Check sheet for the modelled part. Datum: model origin and axes. Units: mm. A direction names the side the tool comes from. Give positions to 0.01 mm unless a question says otherwise; leave off trailing zeros. Write each loop counter-clockwise with the first axis right and the second up, starting at its lowest first coordinate (ties: lowest second). Pieces come first, ordered by that corner, then holes. Notation, with made-up numbers: M 4.5,-32.75 L 63.5,-32.75 A13 cw 63.5,-24.75 Z; hole C 37.5,-9.75 d5. An arc over 180 degrees is marked long. One line per item, written item: value. Start each with the question number.
from build123d import *

# Parameters (mm, degrees)
F1_DEPTH = 15
F2_W     = 50
F2_H     = 32
F3_DEPTH = 150
F4_T     = -2.5


with BuildPart() as f1:
    # F0 (on Top) → F1 (new body)
    with BuildSketch(Plane.XY):
        with BuildLine():
            Line((100, 50), (-100, 50))
            Line((-100, 50), (-100, -50))
            add(Edge.make_bspline(
                [(-100, -50), (-66.6666666667, -68.9898259938), (0, -106.9694779813), (66.6666666667, -68.9898259938), (100, -50)],
                knots=[0, 0, 0, 0, 0.5, 1, 1, 1, 1], degree=3))
            Line((100, -50), (100, 50))
        make_face()
    extrude(amount=F1_DEPTH)

    # F2 (on face) → F3 (join)
    with BuildSketch(Plane.XY.offset(15)):
        with Locations((0, 25.8605617276)):
            Rectangle(F2_W, F2_H)
    extrude(amount=F3_DEPTH)

    # F4
    f4_openings = [f1.faces().sort_by_distance(p)[0] for p in [
        (0, 25.860562, 165),
    ]]
    offset(amount=F4_T, openings=f4_openings, kind=Kind.INTERSECTION)


solid = f1.part
1) Tool access check on faces 1 (the flat face through (0, 39.361, 88)), 2 (the flat face through (-1, -18, 2.5)), 3 (the flat face through (-25, 26, 89)). Record the directions out of +Z, -Z, +X, -X, +Y, -Y that give a thin tool (end or side, any length) a straight path to the whole face; none if there is none.
2) Gauge pin test, flat ends, axial feed: pin 1 (22.5 mm diameter, centred on x = -6.5, z = 73, fed in from +Y); pin 2 (22.5 mm diameter, centred on x = -11, z = 123, fed in from -Y); pin 3 (5 mm diameter, centred on x = -65, y = -68.5, fed in from +Z). Record the tip position at first contact, or that the pin passes through.
3) Cross-section at A-A (z = 95). Record the boundary of the cut face in (x, y), plus the area to 3 significant figures.
4) Material ranges on L1, parallel to Z at x = -58.5, y = -18; L2, parallel to X at y = 36.5, z = 98.5; L3, parallel to X at y = 21.5, z = 11, recorded low to high. Write a range as from..to.
5) Draft check along Y on faces 4 (the flat face through (1, 50, 7)), 5 (the flat face through (25, 26, 89)), 6 (the flat face through (-22.5, 26, 88)), 7 (the flat face through (0, 9.861, 89)). Enter one of: released by +Y, released by -Y, zero draft, split by the parting line, or undercut.
6) Cross-section at B-B (y = 6.5). Record the boundary of the cut face in (x, z).
Data:
1. face 1: +Z
1. face 2: none
1. face 3: +Z, -X, +Y, -Y
2. pin 1: stops at y = 41.86
2. pin 2: stops at y = 9.86
2. pin 3: stops at z = 15
3. outline: M -25,9.86 L 25,9.86 L 25,41.86 L -25,41.86 Z; hole M -22.5,12.36 L 22.5,12.36 L 22.5,39.36 L -22.5,39.36 Z
3. area: 385 mm2
4. L1: z = 0..2.5, 12.5..15
4. L2: x = -25..-22.5, 22.5..25
4. L3: x = -100..-97.5, 97.5..100
5. face 4: released by +Y
5. face 5: zero draft
5. face 6: undercut
5. face 7: released by -Y
6. outline: M -100,0 L 100,0 L 100,15 L -100,15 Z; hole M -97.5,2.5 L 97.5,2.5 L 97.5,12.5 L -97.5,12.5 Z
